Verification items for the finished model (mm, model axes). Face numbers are marked on the shaded views. A direction names the side the tool comes from. Coordinates: 2 decimals unless noted, no trailing zeros. Loops run counter-clockwise (first coordinate to the right, second up) from the corner with the lowest first, then second, coordinate; pieces in that order, holes last. Notation, with made-up numbers: (70, 45) - (79, 45) arc R24 ccw to (79, 56) - close; hole circle Ø10 at (31, 36). An arc over 180 degrees is marked (long way). Answer as CSV lines item,"result". Start each with the question number.
1. Gauge pin test, flat ends, axial feed: P1, Ø1.3, axis at x = 0.5, z = 7, coming from the -Y side; P2, Ø0.8, axis at x = 0.5, z = 8, coming from the +Y side; P3, Ø2, axis at x = 2, z = 8.5, coming from the -Y side. Record the tip position at first contact, or that the pin passes through.
2. Cross-section at A-A (y = 0). Enter the section's corners in (x, z).
3. Release check for a two-part mould opening along Z. For the marked faces 1, 2, 3 and 4 record: pulls with the +Z half, pulls with the -Z half, needs draft (parallel to the pull), parting line crosses it, or undercut.
4. Material ranges on line 1 (Z direction, x = -0.5, y = -3.75); line 2 (Z direction, x = 6.25, y = 2.75); line 3 (X direction, y = 4, z = 10.2), recorded low to high. Write a range as [from, to].
5. Cross-section at B-B (x = 0). Enter the section's corners in (y, z), plus the area to 3 significant figures.
6. Cross-section at C-C (z = 6.7). Enter the section's corners in (x, y) (3 decimals).
7. Set-up check for the marked faces 5, 6 and 7: record each of +Z, -Z, +X, -X, +Y, -Y from which the full face is reachable in a straight line by a thin tool's end or side.
8. Cross-section at D-D (z = 10.4). Enter the section's corners in (x, y).
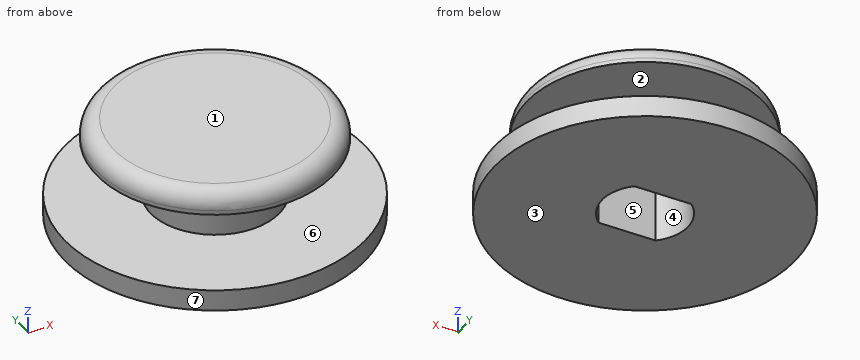
```python
from build123d import *

# Parameters (mm, degrees)
SKETCH006_R     = 7
PAD005_DEPTH    = 1
SKETCH007_R     = 3
PAD006_DEPTH    = 2.7
SKETCH008_R     = 5.5
PAD007_DEPTH    = 1
FILLET_R        = 0.8
POCKET001_DEPTH = 2.7


with BuildPart() as part:
    # Sketch006 → Pad005 (new body)
    with BuildSketch(Plane.XY):
        Circle(SKETCH006_R)
    extrude(amount=PAD005_DEPTH)

    # Sketch007 (on Face3 of Pad005) → Pad006 (join)
    with BuildSketch(Plane.XY.offset(1)):
        Circle(SKETCH007_R)
    extrude(amount=PAD006_DEPTH)

    # Sketch008 (on Face5 of Pad006) → Pad007 (join)
    with BuildSketch(Plane.XY.offset(3.7)):
        Circle(SKETCH008_R)
    extrude(amount=PAD007_DEPTH)

    # Fillet
    fillet_edges = [part.edges().sort_by_distance(p)[0] for p in [
        (-5.5, 0, 4.7),
    ]]
    fillet(fillet_edges, radius=FILLET_R)

    # Sketch009 (on Face8 of Fillet) → Pocket001 (cut)
    with BuildSketch(Plane(origin=(0, 0, 0), x_dir=(1, 0, 0), z_dir=(0, 0, -1))):
        with BuildLine():
            ThreePointArc((-1.325, 1.5), (-2.002124, 0), (-1.325, -1.5))
            Line((-1.325, -1.5), (1.325, -1.5))
            ThreePointArc((1.325, -1.5), (2.002124, 0), (1.325, 1.5))
            Line((-1.325, 1.5), (1.325, 1.5))
        make_face()
    extrude(amount=-POCKET001_DEPTH, mode=Mode.SUBTRACT)


with BuildPart() as part_1:
    # Body003 placement: moved
    add(part.part.moved(Location((0, 0, 6))))


solid = part_1.part
```
Values follow:
1,P1,"stops at y = -7"
1,P2,"stops at y = 3"
1,P3,"stops at y = -2.83"
2,outline,"(-7, 6) - (-2, 6) - (-2, 8.7) - (2, 8.7) - (2, 6) - (7, 6) - (7, 7) - (3, 7) - (3, 9.7) - (5.5, 9.7) - (5.5, 9.9) arc R0.8 ccw to (4.7, 10.7) - (-4.7, 10.7) arc R0.8 ccw to (-5.5, 9.9) - (-5.5, 9.7) - (-3, 9.7) - (-3, 7) - (-7, 7) - close"
3,face 1,"pulls with the +Z half"
3,face 2,"undercut"
3,face 3,"pulls with the -Z half"
3,face 4,"needs draft"
4,line 1,"z = [6, 7], [9.7, 10.7]"
4,line 2,"z = [6, 7]"
4,line 3,"x = [-3.69, 3.69]"
5,outline,"(-7, 6) - (-1.5, 6) - (-1.5, 8.7) - (1.5, 8.7) - (1.5, 6) - (7, 6) - (7, 7) - (3, 7) - (3, 9.7) - (5.5, 9.7) - (5.5, 9.9) arc R0.8 ccw to (4.7, 10.7) - (-4.7, 10.7) arc R0.8 ccw to (-5.5, 9.9) - (-5.5, 9.7) - (-3, 9.7) - (-3, 7) - (-7, 7) - close"
5,area,"32.8 mm²"
6,outline,"circle Ø14 at (0, 0); hole (-1.325, -1.5) - (1.325, -1.5) arc R2 ccw to (1.325, 1.5) - (-1.325, 1.5) arc R2 ccw to start"
7,face 5,"-Z"
7,face 6,"none"
7,face 7,"+Z, -Z"
8,outline,"circle Ø10.65 at (0, 0)"
